Autodesk Fusion 360 part; units mm, degrees
sketch "Sketch1" plane through (0, 0, 0) normal (1, 0, 0) x (0, 1, 0)
  line L0 (-50.7, 0) -> (50.7, 0)
  line L1 (-50.7, 0) -> (-50.7, 15)
  line L2 (-50.7, 15) -> (-54.7, 15)
  line L3 (-54.7, 15) -> (-54.7, -4)
  line L4 (-54.7, -4) -> (54.7, -4)
  line L5 (54.7, -4) -> (54.7, 15)
  line L6 (54.7, 15) -> (50.7, 15)
  line L7 (50.7, 15) -> (50.7, 0)
  dimension "d1" = 101.4
  dimension "d2" = 15
  dimension "d3" = 4
  dimension "d4" = 4
  dimension "d5" = 4
extrude "Extrude1" add sketch "Sketch1" along normal blind 20
sketch "Sketch2" plane through (0, -54.7, 0) normal (0, -1, 0) x (1, 0, 0)
  line L0 (0, 15) -> (0, -4)
  line L1 (0, -4) -> (20, -4)
  line L2 (20, -4) -> (20, 15)
  line L3 (20, 15) -> (0, 15)
  line L4 (7, 12.05) -> (13, 12.05)
  line L5 (3.1, 12.05) -> (16.9, 12.05)
  circle A0 centre (5.05, 12.05) radius 1.95
  circle A1 centre (14.95, 12.05) radius 1.95
  line L6 (10, 12.05) -> (10, 15)
  line L7 (5.05, 14) -> (10, 14)
  dimension "d8" = 6
  dimension "d9" = 13.8
  dimension "d10" = 1
extrude "Extrude2" cut sketch "Sketch2" against normal blind 109.4 contours L5 A1 | L5 A1 | L5 A0 | L5 A0
sketch "Sketch3" plane through (0, 0, 0) normal (0, 0, 1) x (-1, 0, 0)
  line L0 (0, -50.7) -> (0, 50.7)
  line L1 (0, 50.7) -> (-20, 50.7)
  line L2 (-20, 50.7) -> (-20, -50.7)
  line L3 (-20, -50.7) -> (0, -50.7)
  line L4 (0, 0) -> (-20, 0)
  line L5 (-10, 0) -> (-10, -5.6)
  line L6 (-10, 0) -> (-10, -8.4)
  circle A0 centre (-10, -7) radius 1.4
  circle A1 centre (-10, -7) radius 2
  circle A2 centre (-3, 0) radius 2
  circle A3 centre (-10, 7) radius 2
  circle A4 centre (-17, 0) radius 2
  circle A5 centre (-10, 0) radius 3.5
  dimension "d13" = 5.6
  dimension "d14" = 8.4
  dimension "d15" = 4
  dimension "d17" = 360
  dimension "d20" = 7
extrude "Extrude3" cut sketch "Sketch3" against normal blind 4 contours L6 A0 | L6 A0 | A1 | L4 A2 | L4 A2 | L4 A4 | L4 A4 | L4 L5 L6 A5 | L4 A5 | L4 L5 L6 A5 | A3
equation "d13 = ( 11.2 / 2 ) * 1 mm"
equation "d14 = ( 16.8 / 2 ) * 1 mm"
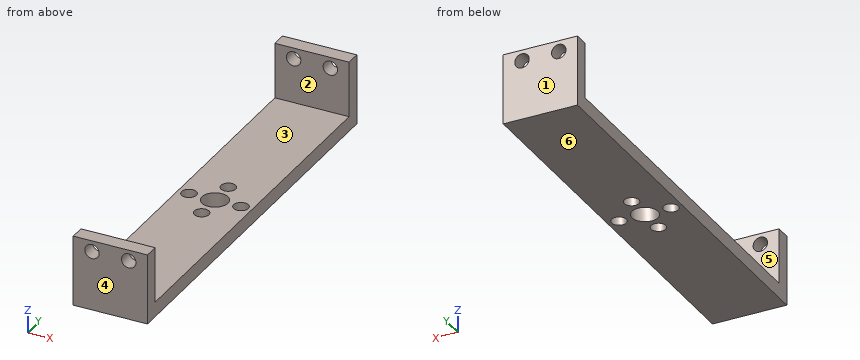
Source: CAD feature listing. Evaluate the final solid. Frame: model axes, mm. Face numbers are marked on the shaded views. A direction names the side the tool comes from. Give positions to 0.01 mm unless a question says otherwise; leave off trailing zeros. Order: outer loops, then holes, each group sorted by start corner. A loop starts at its lowest first (then second) coordinate and runs counter-clockwise, first axis right, second up. Notation, with made-up numbers: (9.5, 58) -> (44.5, 58) arc R22 ccw to (44.5, 83) -> close; hole circle Ø7 at (52, -1.5). An arc over 180 degrees is marked (long way). Use a Markdown table: item, result.
Q1. Section A-A (x = 10). Return the cut outline in (y, z), and give its area (3 significant figures).
A:
| item | result |
|---|---|
| outline | (-54.7, -4) -> (-9, -4) -> (-9, 0) -> (-50.7, 0) -> (-50.7, 15) -> (-54.7, 15) -> close; (-5, -4) -> (-3.5, -4) -> (-3.5, 0) -> (-5, 0) -> close; (3.5, -4) -> (5, -4) -> (5, 0) -> (3.5, 0) -> close; (9, -4) -> (54.7, -4) -> (54.7, 15) -> (50.7, 15) -> (50.7, 0) -> (9, 0) -> close |
| area | 498 mm^2 |
Q2. Section C-C (z = 12.05). Return the cut outline in (x, y).
A:
| item | result |
|---|---|
| outline | (0, -54.7) -> (3.1, -54.7) -> (3.1, -50.7) -> (0, -50.7) -> close; (0, 50.7) -> (3.1, 50.7) -> (3.1, 54.7) -> (0, 54.7) -> close; (7, -54.7) -> (13, -54.7) -> (13, -50.7) -> (7, -50.7) -> close; (7, 50.7) -> (13, 50.7) -> (13, 54.7) -> (7, 54.7) -> close; (16.9, -54.7) -> (20, -54.7) -> (20, -50.7) -> (16.9, -50.7) -> close; (16.9, 50.7) -> (20, 50.7) -> (20, 54.7) -> (16.9, 54.7) -> close |
Q3. Pull-direction query (Y, two-part tool) for the marked faces 3, 4, 5 and 6; classes: +Y half, -Y half, draft (parallel to the pull), parting line (faces both ways), or undercut.
A:
| item | result |
|---|---|
| face 3 | undercut |
| face 4 | -Y half |
| face 5 | undercut |
| face 6 | draft |
Q4. Section B-B (y = 0). Return the cut outline in (x, z), and give its area (3 significant figures).
A:
| item | result |
|---|---|
| outline | (0, -4) -> (1, -4) -> (1, 0) -> (0, 0) -> close; (5, -4) -> (6.5, -4) -> (6.5, 0) -> (5, 0) -> close; (13.5, -4) -> (15, -4) -> (15, 0) -> (13.5, 0) -> close; (19, -4) -> (20, -4) -> (20, 0) -> (19, 0) -> close |
| area | 20.0 mm^2 |
Q5. First-contact query: P1, Ø10, axis at x = 9, y = 0, coming from the +Z side. Flat tip, straight axial feed; report the tip coordinate or a pass-through.
A:
| item | result |
|---|---|
| P1 | z = 0 |
Q6. Access query for the marked faces 1 and 2. Directions: +Z, -Z, +X, -X, +Y, -Y. A direction counts if a zero-diameter tool reaches every point of the face in a straight line with its end or side. Return the directions, or none.
A:
| item | result |
|---|---|
| face 1 | +Z, -Z, +X, -X, +Y |
| face 2 | +Z, +X, -X |
Q7. Material intervals for line 1 (Y direction, x = 10, z = -1.25); line 2 (X direction, y = 0, z = -1); line 3 (Z direction, x = 5.05, y = -52), sorted ascending. Write a range as [from, to].
A:
| item | result |
|---|---|
| line 1 | [-54.7, -9], [-5, -3.5], [3.5, 5], [9, 54.7] |
| line 2 | [0, 1], [5, 6.5], [13.5, 15], [19, 20] |
| line 3 | [-4, 10.1], [14, 15] |
Q8. Section D-D (z = -1.25). Return the cut outline in (x, y), and give its area (3 significant figures).
A:
| item | result |
|---|---|
| outline | (0, -54.7) -> (20, -54.7) -> (20, 54.7) -> (0, 54.7) -> close; hole circle Ø4 at (3, 0); hole circle Ø7 at (10, 0); hole circle Ø4 at (10, -7); hole circle Ø4 at (10, 7); hole circle Ø4 at (17, 0) |
| area | 2,100 mm^2 |
